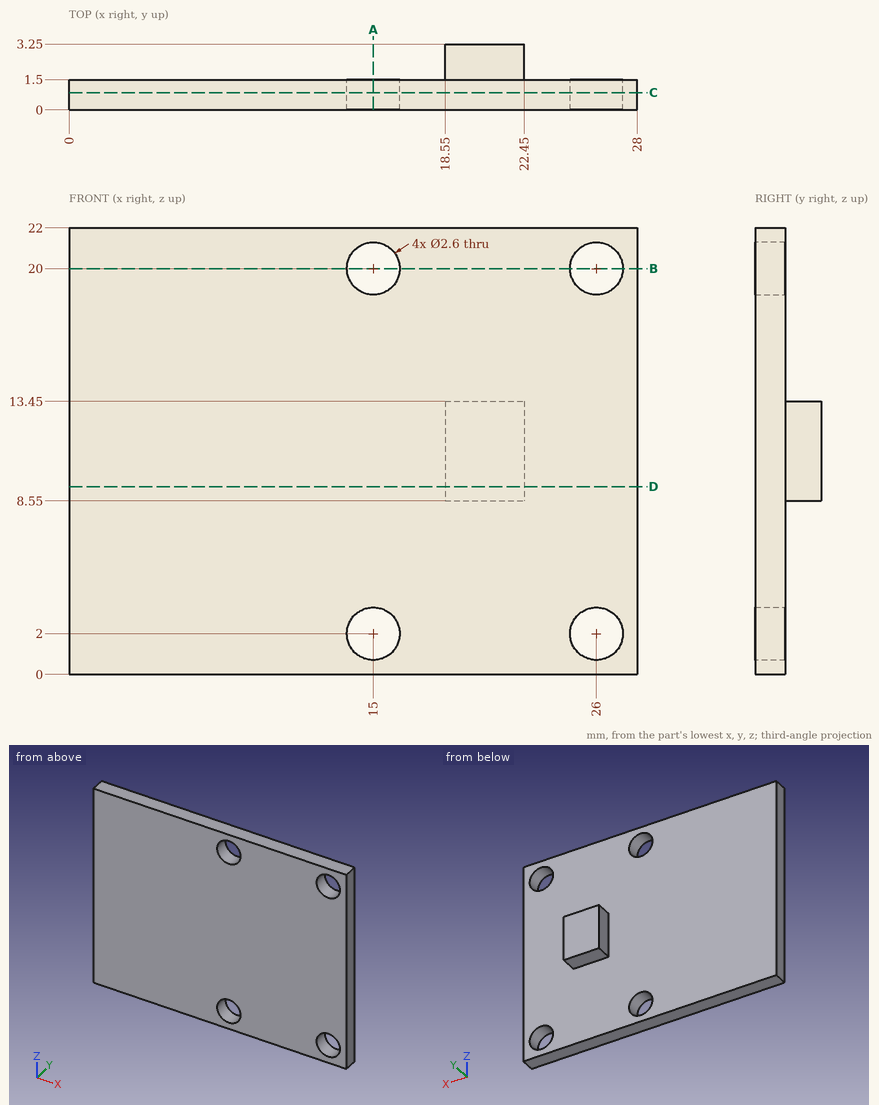
Source: three-view drawing plus pictorial views. Frame: mm from the lowest corner of the part. Give positions to 0.01 mm unless a question says otherwise; leave off trailing zeros. Loops run counter-clockwise (first coordinate to the right, second up) from the corner with the lowest first, then second, coordinate; pieces in that order, holes last.
1) Contact query for flat-ended pins moving along their axis: pin 1 (0.9 mm diameter, centred on y = 2, z = 10, fed in from -X); pin 2 (0.5 mm diameter, centred on x = 21, y = 2.5, fed in from -Z); pin 3 (1.9 mm diameter, centred on x = 21, y = 2.5, fed in from +Z). Output: stop coordinate, or through.
A:
pin 1: stops at x = 18.55
pin 2: stops at z = 8.55
pin 3: stops at z = 13.45
2) Line query: L1, parallel to X at y = 0.95, z = 2; L2, parallel to Y at x = 5, z = 10; L3, parallel to X at y = 2.8, z = 8.75. Output: solid intervals per line, ascending.
A:
L1: x = 0 to 13.7, 16.3 to 24.7, 27.3 to 28
L2: y = 0 to 1.5
L3: x = 18.55 to 22.45
3) Section query D-D on z = 9.25. Return the cut outline in (x, y), and give its area (3 significant figures).
A:
outline: (0, 0) - (28, 0) - (28, 1.5) - (22.45, 1.5) - (22.45, 3.25) - (18.55, 3.25) - (18.55, 1.5) - (0, 1.5) - close
area: 48.8 mm2
4) Section query B-B on z = 20. Return the cut outline in (x, y), and give its area (3 significant figures).
A:
outline: (0, 0) - (13.7, 0) - (13.7, 1.5) - (0, 1.5) - close; (16.3, 0) - (24.7, 0) - (24.7, 1.5) - (16.3, 1.5) - close; (27.3, 0) - (28, 0) - (28, 1.5) - (27.3, 1.5) - close
area: 34.2 mm2
5) Section query C-C on y = 0.85. Return the cut outline in (x, z), and give its area (3 significant figures).
A:
outline: (0, 0) - (28, 0) - (28, 22) - (0, 22) - close; hole circle Ø2.6 at (15, 2); hole circle Ø2.6 at (15, 20); hole circle Ø2.6 at (26, 2); hole circle Ø2.6 at (26, 20)
area: 595 mm2
6) Section query A-A on x = 15. Return the cut outline in (y, z).
A:
outline: (0, 0) - (1.5, 0) - (1.5, 0.7) - (0, 0.7) - close; (0, 3.3) - (1.5, 3.3) - (1.5, 18.7) - (0, 18.7) - close; (0, 21.3) - (1.5, 21.3) - (1.5, 22) - (0, 22) - close
